```python
from build123d import *

# Parameters (mm, degrees)
SKETCH1_R            = 10.5
SKETCH1_R_2          = 5
BOSS_EXTRUDE1_DEPTH  = 10
SKETCH2_R            = 11.62970335
BOSS_EXTRUDE9_DEPTH  = 3
BOSS_EXTRUDE10_DEPTH = 400


with BuildPart() as part:
    # Sketch1 → Boss-Extrude1 (new body)
    # profile 1 of 2: a face of its own
    with BuildSketch(Plane.XY):
        with Locations((-31.363787375, 3.65282392)):
            Circle(SKETCH1_R)
        with Locations((-31.363787375, 3.65282392)):
            Circle(SKETCH1_R_2, mode=Mode.SUBTRACT)
    # profile 2 of 2: a face of its own
    with BuildSketch(Plane.XY):
        with BuildLine():
            Line((-31.363787375, 14.15282392), (-50.863787375, 14.15282392))
            Line((-50.863787375, 14.15282392), (-50.863787375, -6.84717608))
            Line((-50.863787375, -6.84717608), (-31.363787375, -6.84717608))
            ThreePointArc((-31.363787375, -6.84717608), (-41.863787375, 3.65282392), (-31.363787375, 14.15282392))
        make_face()
    extrude(amount=BOSS_EXTRUDE1_DEPTH)

    # Sketch2 → Boss-Extrude9 (add)
    with BuildSketch(Plane.ZY.offset(50.863787375)):
        with Locations(Location((5, 3.65282392, 0), (0, 0, 244.536654938))):
            Circle(SKETCH2_R)
    extrude(amount=BOSS_EXTRUDE9_DEPTH)

    # Sketch2_8 → Boss-Extrude10 (add)
    with BuildSketch(Plane.ZY.offset(50.863787375)):
        with BuildLine():
            ThreePointArc((5, 13.15282392), (2.400826911, 12.790345425), (0, 11.730571131))
            Line((0, 11.730571131), (0, 9.897821919))
            ThreePointArc((0, 9.897821919), (2.350470229, 11.201333177), (5, 11.65282392))
            Line((5, 11.65282392), (5, 13.15282392))
        make_face()
        with BuildLine():
            Line((0, -2.592174078), (0, -4.42492329))
            ThreePointArc((0, -4.42492329), (2.400826911, -5.484697585), (5, -5.84717608))
            Line((5, -5.84717608), (5, -4.34717608))
            ThreePointArc((5, -4.34717608), (2.350470229, -3.895685336), (0, -2.592174078))
        make_face()
        with BuildLine():
            ThreePointArc((10, 11.730571131), (7.599173089, 12.790345425), (5, 13.15282392))
            Line((5, 13.15282392), (5, 11.65282392))
            ThreePointArc((5, 11.65282392), (7.649529771, 11.201333177), (10, 9.897821919))
            Line((10, 9.897821919), (10, 11.730571131))
        make_face()
        with BuildLine():
            ThreePointArc((5, -5.84717608), (7.599173089, -5.484697585), (10, -4.42492329))
            Line((10, -4.42492329), (10, -2.592174078))
            ThreePointArc((10, -2.592174078), (7.649529771, -3.895685336), (5, -4.34717608))
            Line((5, -4.34717608), (5, -5.84717608))
        make_face()
        with BuildLine():
            ThreePointArc((14.5, 3.65282392), (13.299096336, 8.276134422), (10, 11.730571131))
            Line((10, 11.730571131), (10, 9.897821919))
            ThreePointArc((10, 9.897821919), (12.211102551, 7.116925535), (13, 3.65282392))
            ThreePointArc((13, 3.65282392), (12.211102551, 0.188722305), (10, -2.592174078))
            Line((10, -2.592174078), (10, -4.42492329))
            ThreePointArc((10, -4.42492329), (13.299096336, -0.970486582), (14.5, 3.65282392))
        make_face()
        with BuildLine():
            Line((0, 9.897821919), (0, 11.730571131))
            ThreePointArc((0, 11.730571131), (-4.5, 3.65282392), (0, -4.42492329))
            Line((0, -4.42492329), (0, -2.592174078))
            ThreePointArc((0, -2.592174078), (-3, 3.65282392), (0, 9.897821919))
        make_face()
    extrude(amount=BOSS_EXTRUDE10_DEPTH)


solid = part.part
```
Part model, mm, in its own coordinate system. A direction names the side the tool comes from. Coordinates: 2 decimals unless noted, no trailing zeros. Order: outer loops, then holes, each group sorted by start corner. A loop starts at its lowest first (then second) coordinate and runs counter-clockwise, first axis right, second up. Notation, with made-up numbers: (-26, 50) - (5, 50) arc R23 ccw to (5, 66) - close; hole circle Ø3 at (14, 8). An arc over 180 degrees is marked (long way). Return JSON: item names as keys, results as strings. Group by question number.
Item 1: Cut at A-A (x = -353). List the corners of the cut face in (y, z).
Item 2: Pull direction Z, two halves, no side cores. Call faces 5 (the face through (-53.864, 4, 5)), 6 (the face through (-39, 4, 10)), 7 (the face through (-52.343, -6.208, 11.166)), 8 (the face through (-450.864, -3, 0)): pulls with the +Z half, pulls with the -Z half, needs draft (parallel to the pull), parting line crosses it, or undercut.
Item 3: Drill centre lines: probe 1 along Z at (x, y) = (-174.5, 4.5); probe 2 along X at (y, z) = (3.5, 11); probe 3 along Z at (x, y) = (-223.5, -2.25). Where is each one in solid material? Low to high. Write a range as from..to.
Item 4: Which spindle directions (+Z, -Z, +X, -X, +Y, -Y) get a long thin tool onto all of the face, cutting with end or side? Do faces 1 (the face through (-41, 14.153, 5)), 2 (the face through (-39, 4, 0)), 3 (the face through (-50.864, 3, 12)), 4 (the face through (-53.864, 11.3, -0.9)). Say none if no direction does.
Item 5: Pin check, flat tips, straight feed: pin 1 (8 mm diameter, centred on y = 12, z = 10.5, fed in from +X); pin 2 (4 mm diameter, centred on x = -160.5, y = 9, fed in from -Z); pin 3 (4 mm diameter, centred on y = -3, z = 14, fed in from +X). Stop position of each tip, or through.
Check values:
{
 "1": {"outline": "circle Ø19 at (3.65, 5); hole circle Ø16 at (3.65, 5)"},
 "2": {"face 5": "undercut", "face 6": "pulls with the +Z half", "face 7": "parting line crosses it", "face 8": "needs draft"},
 "3": {"probe 1": "z = -4.46..-2.96, 12.96..14.46", "probe 2": "x = -53.86..-50.86", "probe 3": "z = -2.44..-0.4, 10.4..12.44"},
 "4": {"face 1": "+Z, -Z, +X, +Y", "face 2": "-Z, +X, +Y, -Y", "face 3": "+Z, +X, +Y, -Y", "face 4": "-X"},
 "5": {"pin 1": "stops at x = -21.82", "pin 2": "stops at z = -3.89", "pin 3": "stops at x = -50.86"}
}
